Verification items for the finished model (mm, model axes). Face numbers are marked on the shaded views. A direction names the side the tool comes from. Coordinates: 2 decimals unless noted, no trailing zeros. Write each loop counter-clockwise with the first axis right and the second up, starting at its lowest first coordinate (ties: lowest second). Pieces come first, ordered by that corner, then holes. Notation, with made-up numbers: (-29, 0.5) -> (21, 0.5) arc R16 cw to (21, 11.5) -> close; hole circle Ø7 at (39.25, -33.5). An arc over 180 degrees is marked (long way). Answer in a Markdown table with one row per item.
```python
from build123d import *

# Parameters (mm, degrees)
SKETCH_R     = 4
PAD_DEPTH    = 5
POCKET_DEPTH = 2


with BuildPart() as part:
    # Sketch → Pad (new body)
    with BuildSketch(Plane.XY):
        with BuildLine():
            Line((-15, -9.5), (15, -9.5))
            ThreePointArc((15, -9.5), (19.242641, -7.742641), (21, -3.5))
            Line((21, -3.5), (21, 3.5))
            ThreePointArc((21, 3.5), (19.242641, 7.742641), (15, 9.5))
            Line((15, 9.5), (-15, 9.5))
            ThreePointArc((-15, 9.5), (-19.242641, 7.742641), (-21, 3.5))
            Line((-21, 3.5), (-21, -3.5))
            ThreePointArc((-21, -3.5), (-19.242641, -7.742641), (-15, -9.5))
        make_face()
        Circle(SKETCH_R, mode=Mode.SUBTRACT)
        with BuildLine():
            ThreePointArc((-12, 3.5), (-15, 6.5), (-18, 3.5))
            Line((-18, 3.5), (-18, -3.5))
            ThreePointArc((-18, -3.5), (-15, -6.5), (-12, -3.5))
            Line((-12, 3.5), (-12, -3.5))
        make_face(mode=Mode.SUBTRACT)
        with BuildLine():
            ThreePointArc((18, 3.5), (15, 6.5), (12, 3.5))
            Line((12, 3.5), (12, -3.5))
            ThreePointArc((12, -3.5), (15, -6.5), (18, -3.5))
            Line((18, 3.5), (18, -3.5))
        make_face(mode=Mode.SUBTRACT)
    extrude(amount=PAD_DEPTH)

    # Sketch001 (on Face19 of Pad) → Pocket (cut)
    with BuildSketch(Plane.XY.offset(5)):
        Polygon((6.5, 3.752777), (0, 7.505553), (-6.5, 3.752777), (-6.5, -3.752777), (0, -7.505553), (6.5, -3.752777), align=None)
    extrude(amount=-POCKET_DEPTH, mode=Mode.SUBTRACT)


solid = part.part
```
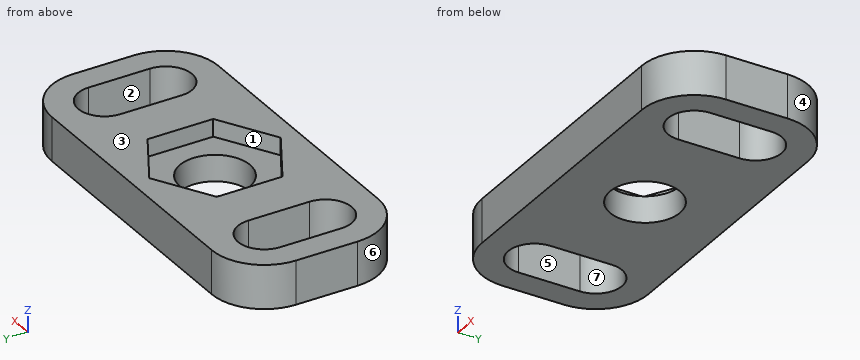
1. Sectioned sample at C-C, the plane y = -5. Record the cut outline in (x, z), and give its area (3 significant figures).
Findings below:
| item | result |
|---|---|
| outline | (-20.81, 0) -> (-17.6, 0) -> (-17.6, 5) -> (-20.81, 5) -> close; (-12.4, 0) -> (12.4, 0) -> (12.4, 5) -> (4.34, 5) -> (4.34, 3) -> (-4.34, 3) -> (-4.34, 5) -> (-12.4, 5) -> close; (17.6, 0) -> (20.81, 0) -> (20.81, 5) -> (17.6, 5) -> close |
| area | 139 mm² |
2. Sectioned sample at D-D, the plane x = -3.5. Record the cut outline in (y, z), and give its area (3 significant figures).
Findings below:
| item | result |
|---|---|
| outline | (-9.5, 0) -> (-1.94, 0) -> (-1.94, 3) -> (-5.48, 3) -> (-5.48, 5) -> (-9.5, 5) -> close; (1.94, 0) -> (9.5, 0) -> (9.5, 5) -> (5.48, 5) -> (5.48, 3) -> (1.94, 3) -> close |
| area | 61.4 mm² |
3. Material ranges on probe 1 along X at (y, z) = (0, 1.9); probe 2 along X at (y, z) = (1, 3.25); probe 3 along Y at (x, z) = (0, 1.1), recorded low to high. Write a range as from..to.
Findings below:
| item | result |
|---|---|
| probe 1 | x = -21..-18, -12..-4, 4..12, 18..21 |
| probe 2 | x = -21..-18, -12..-6.5, 6.5..12, 18..21 |
| probe 3 | y = -9.5..-4, 4..9.5 |
4. Sectioned sample at A-A, the plane y = 0. Record the cut outline in (x, z).
Findings below:
| item | result |
|---|---|
| outline | (-21, 0) -> (-18, 0) -> (-18, 5) -> (-21, 5) -> close; (-12, 0) -> (-4, 0) -> (-4, 3) -> (-6.5, 3) -> (-6.5, 5) -> (-12, 5) -> close; (4, 0) -> (12, 0) -> (12, 5) -> (6.5, 5) -> (6.5, 3) -> (4, 3) -> close; (18, 0) -> (21, 0) -> (21, 5) -> (18, 5) -> close |
5. Go/stop test with flat-tipped pins: pin 1 (3 mm diameter, centred on y = -5.5, z = 1.5, fed in from -X); pin 2 (7 mm diameter, centred on x = 0, y = 0, fed in from +Z). Record where each tip stops, or that it passes through.
Findings below:
| item | result |
|---|---|
| pin 1 | stops at x = -20.98 |
| pin 2 | passes through |
6. Release check for a two-part mould opening along X. For the marked faces 4, 5, 6 and 7 record: released by +X, released by -X, zero draft, split by the parting line, or undercut.
Findings below:
| item | result |
|---|---|
| face 4 | released by +X |
| face 5 | undercut |
| face 6 | released by -X |
| face 7 | undercut |
7. Access from +Z, -Z, +X, -X, +Y, -Y to the whole of each face (thin tool, end or side, straight path). Record for the marked faces 1, 2 and 3.
Findings below:
| item | result |
|---|---|
| face 1 | +Z |
| face 2 | +Z, -Z |
| face 3 | +Z, +X, -X, +Y, -Y |
8. Sectioned sample at B-B, the plane z = 4. Record the cut outline in (x, y).
Findings below:
| item | result |
|---|---|
| outline | (-21, -3.5) arc R6 ccw to (-15, -9.5) -> (15, -9.5) arc R6 ccw to (21, -3.5) -> (21, 3.5) arc R6 ccw to (15, 9.5) -> (-15, 9.5) arc R6 ccw to (-21, 3.5) -> close; hole (-18, -3.5) arc R3 ccw to (-12, -3.5) -> (-12, 3.5) arc R3 ccw to (-18, 3.5) -> close; hole (-6.5, -3.75) -> (0, -7.51) -> (6.5, -3.75) -> (6.5, 3.75) -> (0, 7.51) -> (-6.5, 3.75) -> close; hole (12, -3.5) arc R3 ccw to (18, -3.5) -> (18, 3.5) arc R3 ccw to (12, 3.5) -> close |
